from build123d import *

# Parameters (mm, degrees)
SKETCH_1_W          = 20
SKETCH_1_H          = 25
EXTRUDE_1_DEPTH     = 15
SKETCH_2_W          = 18
SKETCH_2_H          = 7
SKETCH_2_H_2        = 15
CUT_EXTRUDE_1_DEPTH = 14
SKETCH_5_R          = 0.4
FILLET_1_R          = 1
SKETCH_7_R          = 0.25
EXTRUDE_3_DEPTH     = 1
FILLET_2_R          = 0.2


with BuildPart() as part:
    # 草圖1 → 填料-伸長1 (new body)
    with BuildSketch(Plane.XY):
        Rectangle(SKETCH_1_W, SKETCH_1_H)
    extrude(amount=EXTRUDE_1_DEPTH)

    # 草圖2 → 除料-伸長1 (cut)
    with BuildSketch(Plane.XY.offset(15)):
        with Locations((0, 8)):
            Rectangle(SKETCH_2_W, SKETCH_2_H)
        with Locations((0, -4)):
            Rectangle(SKETCH_2_W, SKETCH_2_H_2)
    extrude(amount=-CUT_EXTRUDE_1_DEPTH, mode=Mode.SUBTRACT)

    # 草圖4 → 旋轉4 (revolve)
    with BuildSketch(Plane(origin=(0, 0, 0), x_dir=(0, 0, -1), z_dir=(1, 0, 0)), mode=Mode.PRIVATE) as revolve_4_sk:
        with BuildLine():
            Line((-15, 16.5), (-14.680951103, 16.5))
            ThreePointArc((-14.680951103, 16.5), (-12.457373104, 13.7185354), (-9.016987566, 12.799518652))
            Line((-9.016987566, 12.799518652), (-9, 12.799518652))
            Line((-9, 12.799518652), (-9, 12.5))
            ThreePointArc((-9, 12.5), (-12.66795249, 13.498071265), (-15, 16.5))
        make_face()
    revolve(revolve_4_sk.sketch.rotate(Axis((0, -12.5, 9), (0, 1, 0)), 90), axis=Axis((0, -12.5, 9), (0, 1, 0)))

    # 掃出1: sweep along a path in 草圖6
    with BuildLine(Plane(origin=(0, 0, 0), x_dir=(0, 0, -1), z_dir=(1, 0, 0))) as sweep_1_path:
        Line((-1.7, 12.5), (-1.7, 20.5))
        ThreePointArc((-1.7, 20.5), (-3.443337751, 23.224114533), (-6.647199994, 22.782194598))
        ThreePointArc((-6.647199994, 22.782194598), (-6.906171507, 22.440350482), (-6.998133329, 22.021463065))
        Line((-6.998133329, 22.021463065), (-6.998133329, 21.428362829))
    # 草圖5 → 掃出1 (sweep)
    with BuildSketch(Plane(origin=(0, 12.5, 0), x_dir=(1, 0, 0), z_dir=(0, 1, 0))):
        with Locations((0, -1.7)):
            Circle(SKETCH_5_R)
    sweep(path=sweep_1_path.line)

    # 圓角1
    fillet_1_edges = [part.edges().sort_by_distance(p)[0] for p in [
        (-0.4, 12.5, 1.7),
    ]]
    fillet(fillet_1_edges, radius=FILLET_1_R)

    # 草圖7 → 填料-伸長3 (add)
    with BuildSketch(Plane(origin=(0, 0, 0), x_dir=(0, 0, -1), z_dir=(1, 0, 0))):
        with Locations(Location((-1.7, 18.8, 0), (0, 0, 270))):
            Circle(SKETCH_7_R)
    extrude(amount=EXTRUDE_3_DEPTH)

    # 草圖8 → 旋轉5 (revolve)
    with BuildSketch(Plane(origin=(1, 0, 0), x_dir=(0, 0, -1), z_dir=(1, 0, 0))):
        Polygon((-2.619253332, 19.571345132), (-1.7, 18.8), (-1.73213938, 18.761697778), (-2.651392712, 19.533042909), align=None)
    revolve(axis=Axis((1, 18.8, 1.7), (0, -0.6427876096865434, -0.7660444431189747)))

    # 圓角2
    fillet_2_edges = [part.edges().sort_by_distance(p)[0] for p in [
        (-0.4, 21.428362829, 6.998133329),
    ]]
    fillet(fillet_2_edges, radius=FILLET_2_R)


solid = part.part
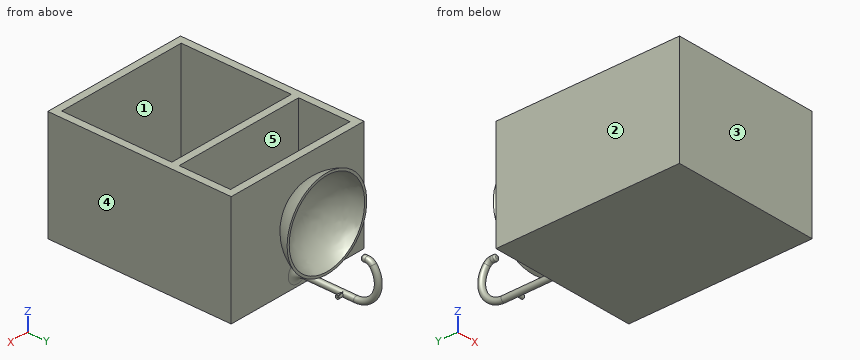
Read the model definition and answer for the solid it produces. Units are mm, in the model's axes. Face numbers are marked on the shaded views. A direction names the side the tool comes from. Give positions to 0.01 mm unless a question says otherwise; leave off trailing zeros. Write each loop counter-clockwise with the first axis right and the second up, starting at its lowest first coordinate (ties: lowest second). Pieces come first, ordered by that corner, then holes. Notation, with made-up numbers: (-20, 54.25) - (-12, 54.25) arc R14 ccw to (-12, 75.25) - close; hole circle Ø9 at (16.5, 52). An arc over 180 degrees is marked (long way). Return JSON: item names as keys, results as strings.
Q1. For a pull along Y with two mould halves and no side action, classify the marked faces 3, 4 and 5 as released by +Y, released by -Y, zero draft, split by the parting line, or undercut.
Reply:
{"face 3": "released by -Y", "face 4": "zero draft", "face 5": "undercut"}
Q2. A cutting plane is placed at B-B, the plane y = -9.5. Determine the outline of the cut face in (x, z), and give its area (3 significant figures).
Reply:
{"outline": "(-10, 0) - (10, 0) - (10, 15) - (9, 15) - (9, 1) - (-9, 1) - (-9, 15) - (-10, 15) - close", "area": "48.0 mm²"}
Q3. A cutting plane is placed at C-C, the plane z = 13. Count the separate pieces of the cut face and the enclosed holes in it, and give its area (3 significant figures).
Reply:
{"separate pieces": "2", "enclosed holes": "2", "area": "108 mm²"}
Q4. For the marked faces 1 and 2, determine the directions among +Z, -Z, +X, -X, +Y, -Y from which every point of the face is accessible in a straight line to the end or side of a thin tool.
Reply:
{"face 1": "+Z", "face 2": "+Z, -Z, -X, +Y, -Y"}
Q5. Consider line 1 along Y through (x, z) = (8.5, 5); line 2 along X through (y, z) = (-8, 13); line 3 along Y through (x, z) = (-3.25, 12.5). Determine where each line is inside the solid, lowest interval first. Write a range as [from, to].
Reply:
{"line 1": "[-12.5, -11.5], [3.5, 4.5], [11.5, 12.5]", "line 2": "[-10, -9], [9, 10]", "line 3": "[-12.5, -11.5], [3.5, 4.5], [11.5, 12.5], [14.45, 14.91]"}
Q6. A cutting plane is placed at A-A, the plane x = 7. Determine the outline of the cut face in (y, z), and give its area (3 significant figures).
Reply:
{"outline": "(-12.5, 0) - (12.5, 0) - (12.5, 15) - (11.5, 15) - (11.5, 1) - (4.5, 1) - (4.5, 15) - (3.5, 15) - (3.5, 1) - (-11.5, 1) - (-11.5, 15) - (-12.5, 15) - close", "area": "67.0 mm²"}
Q7. Given P1, Ø4, axis at x = 4.5, z = 2, coming from the +Y side; P2, Ø4, axis at x = 6.5, z = 8.5, coming from the +Y side, each flat-ended and moving along its own axis, determine where each tip first touches the part or whether it passes through.
Reply:
{"P1": "y = 12.5", "P2": "y = 16.5"}
